Could you check a few things on this drawing? It's one solid part, dimensions in mm from its lowest x, y, z. A direction names the side the tool comes from. Give positions to 0.01 mm unless a question says otherwise; leave off trailing zeros. Order: outer loops, then holes, each group sorted by start corner. A loop starts at its lowest first (then second) coordinate and runs counter-clockwise, first axis right, second up.
Item 1: If we mould it in two halves opening along X, with no side actions, what happens to the marked faces 4, 5, 6 and 7? For each: +X half, -X half, draft (parallel to the pull), parting line (faces both ways), or undercut.
Item 2: I want a section at A-A, the plane z = 2.55. Write out the boundary of the cut face in (x, y).
Item 3: I want a section at C-C, the plane x = 20. Write out the boundary of the cut face in (y, z), then the cut area to 3 significant figures.
Item 4: I want a section at B-B, the plane y = 6. Write out the boundary of the cut face in (x, z), then the cut area to 3 significant figures.
Item 5: I want a section at D-D, the plane y = 38. Write out the boundary of the cut face in (x, z), then the cut area to 3 significant figures.
Item 6: If I drill on line 1 along Y through (x, z) = (11, 0.85); line 2 along Z through (x, y) = (8.4, 42.5); line 3 along Y through (x, z) = (20, 3.1), over which ranges is the centre line in solid material (lowest first)?
Item 7: Which directions (+Z, -Z, +X, -X, +Y, -Y) give clear straight access to the entire face, cutting with the end or side of a thin tool? Please do the marked faces 1, 2 and 3.
Item 8: I'm going to push flat-ended pins straight in: pin 1 Ø1.5 at (x, z) = (27.5, 2) entering from +Y; pin 2 Ø2.5 at (x, z) = (35, 2.5) entering from +Y; pin 3 Ø1.5 at (y, z) = (33.5, 1.5) entering from +X. Where does each tip first touch, or does it pass through?
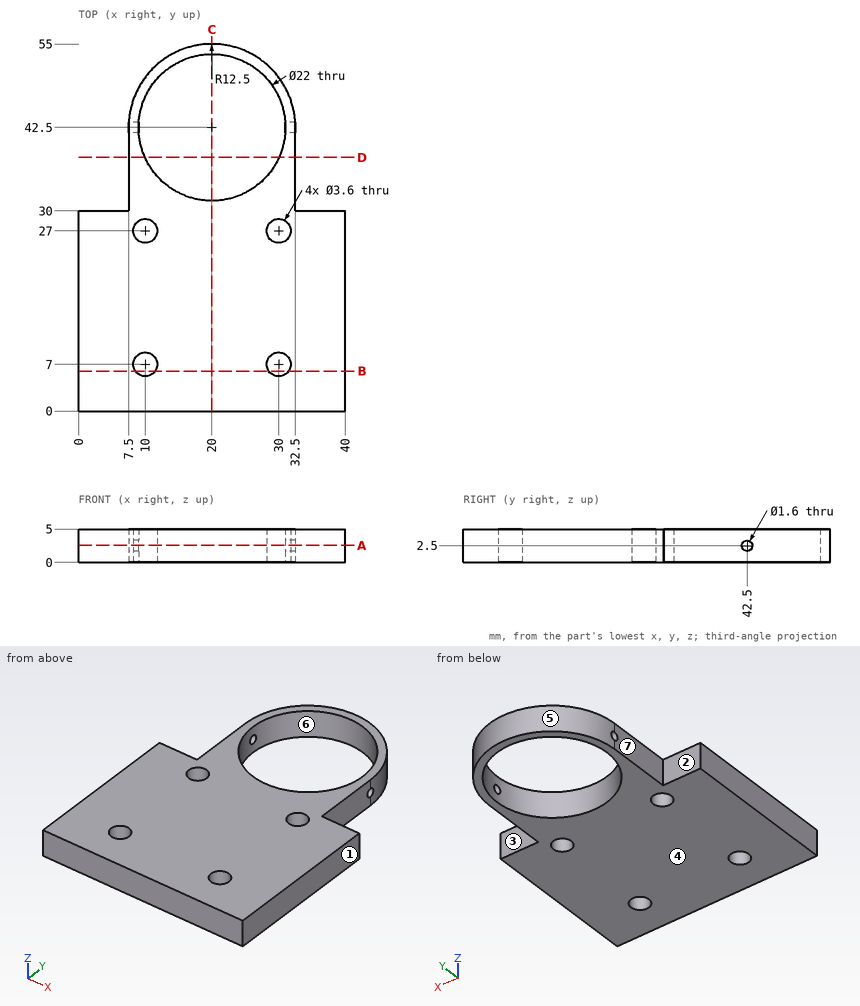
Results list:
1. face 4: draft
1. face 5: parting line
1. face 6: undercut
1. face 7: -X half
2. outline: (0, 0) - (40, 0) - (40, 30) - (32.5, 30) - (32.5, 41.7) - (30.97, 41.7) arc R11 cw to (9.03, 41.7) - (7.5, 41.7) - (7.5, 30) - (0, 30) - close; (7.53, 43.3) - (9.03, 43.3) arc R11 cw to (30.97, 43.3) - (32.47, 43.3) arc R12.5 ccw to start; hole circle Ø3.6 at (10, 7); hole circle Ø3.6 at (10, 27); hole circle Ø3.6 at (30, 7); hole circle Ø3.6 at (30, 27)
3. outline: (0, 0) - (31.5, 0) - (31.5, 5) - (0, 5) - close; (53.5, 0) - (55, 0) - (55, 5) - (53.5, 5) - close
3. area: 165 mm2
4. outline: (0, 0) - (8.5, 0) - (8.5, 5) - (0, 5) - close; (11.5, 0) - (28.5, 0) - (28.5, 5) - (11.5, 5) - close; (31.5, 0) - (40, 0) - (40, 5) - (31.5, 5) - close
4. area: 170 mm2
5. outline: (7.5, 0) - (9.96, 0) - (9.96, 5) - (7.5, 5) - close; (30.04, 0) - (32.5, 0) - (32.5, 5) - (30.04, 5) - close
5. area: 24.6 mm2
6. line 1: y = 0 to 5.5, 8.5 to 25.5, 28.5 to 36.18, 48.82 to 51.17
6. line 2: z = 0 to 1.7, 3.3 to 5
6. line 3: y = 0 to 31.5, 53.5 to 55
7. face 1: +Z, -Z, +X, +Y, -Y
7. face 2: +Z, -Z, -X, +Y
7. face 3: +Z, -Z, +X, +Y
8. pin 1: stops at y = 53.02
8. pin 2: stops at y = 30
8. pin 3: stops at x = 32.5
